Here's how the part is built. I have some questions about the finished solid (model axes, mm). A direction names the side the tool comes from. Round coordinates to 2 decimals unless told otherwise and drop trailing zeros. Loops run counter-clockwise (first coordinate to the right, second up) from the corner with the lowest first, then second, coordinate; pieces in that order, holes last. Notation, with made-up numbers: M 36,9 L 89,9 A26 ccw 89,45 Z; hole C 24.25,-28 d10. An arc over 180 degrees is marked long. Use a Markdown table: item, result.
Autodesk Inventor part; units mm, degrees
ref_plane "YZ Plane" through (0, 0, 0) normal (1, 0, 0) x (0, 1, 0)
ref_plane "XZ Plane" through (0, 0, 0) normal (0, 1, 0) x (-1, 0, 0)
ref_plane "XY Plane" through (0, 0, 0) normal (0, 0, 1) x (1, 0, 0)
sketch "スケッチ1" plane through (0, 0, 0) normal (0, 1, 0) x (-1, 0, 0)
  line L0 (0, 0) -> (53.8, 0)
  line L1 (53.8, 0) -> (53.8, -71.8)
  line L2 (53.8, -71.8) -> (0, -71.8)
  line L3 (0, -71.8) -> (0, 0)
  dimension "d0" = 53.8
  dimension "d1" = 71.8
extrude "押し出し1" add sketch "スケッチ1" along normal blind 10
sketch "スケッチ2" plane through (0, 10, 0) normal (0, 1, 0) x (1, 0, 0)
  line L0 (-53.8, 71.8) -> (-53.8, 0)
  line L1 (-53.8, 0) -> (0, 0)
  line L2 (-26.9, 0) -> (-26.9, 71.8)
  line L3 (0, 71.8) -> (-53.8, 71.8)
  line L4 (-53.8, 35.9) -> (0, 35.9)
  line L5 (0, 0) -> (0, 71.8)
  line L6 (-26.9, 35.9) -> (-37.05, 35.9)
  line L7 (-37.05, 35.9) -> (-37.05, 56.05)
  line L8 (-37.05, 56.05) -> (-26.9, 56.05)
  line L9 (-26.9, 56.05) -> (-26.9, 35.9)
  line L10 (-37.05, 35.9) -> (-37.05, 15.75)
  line L11 (-37.05, 15.75) -> (-26.9, 15.75)
  line L12 (-16.75, 35.9) -> (-16.75, 56.05)
  line L13 (-16.75, 56.05) -> (-26.9, 56.05)
  line L14 (-16.75, 35.9) -> (-16.75, 15.75)
  line L15 (-16.75, 15.75) -> (-26.9, 15.75)
  dimension "d7" = 20.15
  dimension "d8" = 10.15
extrude "押し出し2" add sketch "スケッチ2" along normal blind 40 contours L3 L2 L8 L7 L4 L0 | L4 L10 L11 L2 L1 L0 | L3 L5 L4 L12 L13 L2 | L2 L15 L14 L4 L5 L1
fillet "フィレット1" radius 5 4 edges at (0, 25, 0) (0, 25, -71.8) (-53.8, 25, -71.8) (-53.8, 25, 0)
sketch "スケッチ3" plane through (0, 0, -5) normal (1, 0, 0) x (0, 0, -1)
  line L0 (51.05, 50) -> (10.75, 50)
  line L1 (30.9, 50) -> (30.9, 0)
  line L2 (0, 0) -> (61.8, 0)
  line L3 (20.9, 50) -> (20.9, 0)
  line L4 (0, 50) -> (0, 0)
  line L5 (0, 10) -> (62, 10)
  line L6 (10.75, 10) -> (51.05, 10)
  point P0 (-5, 0)
  point P1 (20.9, 20)
  point P2 (20.9, 40)
  point P3 (40.9, 20)
  point P4 (40.9, 40)
  dimension "d12" = 10
  dimension "d13" = 10
  dimension "d14" = 10
  dimension "d15" = 20
hole "穴1" at (0, 20, -25.9) at (0, 40, -25.9) at (0, 40, -45.9) at (0, 20, -45.9) direction (-1, 0, 0) diameter 3.3 end through all
sketch "スケッチ4" plane through (0, 0, 0) normal (0, -1, 0) x (1, 0, 0)
  line L0 (-5, -71.8) -> (-48.8, -71.8)
  line L1 (-26.9, -71.8) -> (-26.9, 0)
  line L2 (-48.8, 0) -> (-5, 0)
  line L3 (-53.8, -66.8) -> (-53.8, -5)
  line L4 (-53.8, -35.9) -> (0, -35.9)
  line L5 (0, -5) -> (0, -66.8)
  point P0 (0, 0)
  point P1 (-26.9, -45.9)
  point P2 (-26.9, -25.9)
  dimension "d23" = 10
  dimension "d24" = 10
hole "穴2" at (-26.9, 0, -45.9) at (-26.9, 0, -25.9) direction (0, 1, 0) diameter 4.1 end through all
fillet "フィレット2" radius 1 4 edges at (-37.05, 50, -35.9) (-26.9, 50, -15.75) (-16.75, 50, -35.9) (-26.9, 50, -56.05)
sketch "スケッチ5" plane through (0, 0, 0) normal (0, -1, 0) x (1, 0, 0)
  circle A0 centre (-26.9, -25.9) radius 2.05
  circle A1 centre (-26.9, -45.9) radius 2.05
  line L0 (-26.9, -25.9) -> (-26.9, -45.9)
  line L1 (-26.9, -35.9) -> (-17.9, -35.9)
  line L2 (-17.9, -35.9) -> (-17.9, -42.9)
  line L3 (-17.9, -42.9) -> (-26.9, -42.9)
  line L4 (-26.9, -42.9) -> (-26.9, -35.9)
  line L5 (-17.9, -35.9) -> (-17.9, -28.9)
  line L6 (-17.9, -28.9) -> (-26.9, -28.9)
  line L7 (-35.9, -35.9) -> (-35.9, -42.9)
  line L8 (-35.9, -42.9) -> (-26.9, -42.9)
  line L9 (-35.9, -35.9) -> (-35.9, -28.9)
  line L10 (-35.9, -28.9) -> (-26.9, -28.9)
  point P0 (0, 0)
  dimension "d33" = 7
  dimension "d34" = 9
extrude "押し出し3" cut sketch "スケッチ5" against normal blind 10 contours L6 L5 L1 L0 | L0 L8 L7 L9 L10 | L1 L2 L3 L0
properties part number "framefixpart1"
1. Imagine slicing it at C-C, the plane y = 44. Write out the boundary of the cut face in (x, z), then the cut area to 3 significant figures.
Answer sheet:
| item | result |
|---|---|
| outline | M -53.8,-66.8 A5 ccw -48.8,-71.8 L -5,-71.8 A5 ccw 0,-66.8 L 0,-5 A5 ccw -5,0 L -48.8,0 A5 ccw -53.8,-5 Z; hole M -37.05,-56.05 L -16.75,-56.05 L -16.75,-15.75 L -37.05,-15.75 Z |
| area | 3,020 mm2 |
2. For pin 1 Ø3.5 at (x, z) = (-26.9, -45.9) entering from +Y; pin 2 Ø16 at (x, z) = (-25, -33.5) entering from +Y, each with a flat end and sliding along its axis, tell me the tip position at first contact or that it passes through.
Answer sheet:
| item | result |
|---|---|
| pin 1 | through |
| pin 2 | y = 10 |
3. Imagine slicing it at B-B, the plane x = -23. Write out the boundary of the cut face in (y, z), then the cut area to 3 significant figures.
Answer sheet:
| item | result |
|---|---|
| outline | M 0,-71.8 L 50,-71.8 L 50,-57.05 A1 ccw 49,-56.05 L 10,-56.05 L 10,-42.9 L 0,-42.9 Z; M 0,-28.9 L 10,-28.9 L 10,-15.75 L 49,-15.75 A1 ccw 50,-14.75 L 50,0 L 0,0 Z |
| area | 1,840 mm2 |
4. Imagine slicing it at A-A, the plane z = -45.9. State how many separate pieces and enclosed holes the cut face has, then the cut area to 3 significant figures.
Answer sheet:
| item | result |
|---|---|
| separate pieces | 6 |
| enclosed holes | 0 |
| area | 1,620 mm2 |
5. Which directions (+Z, -Z, +X, -X, +Y, -Y) give clear straight access to the entire face, cutting with the end or side of a thin tool? Please do faces 5 (the face through (-53.8, 25, -35)), 6 (the face through (-17.7, 10, -35.6)), 7 (the face through (-17.9, 5, -36)).
Answer sheet:
| item | result |
|---|---|
| face 5 | +Z, -Z, -X, +Y, -Y |
| face 6 | +Y |
| face 7 | +Y, -Y |
6. Imagine slicing it at D-D, the plane z = -30. Write out the boundary of the cut face in (x, y).
Answer sheet:
| item | result |
|---|---|
| outline | M -53.8,0 L -35.9,0 L -35.9,10 L -37.05,10 L -37.05,49 A1 ccw -38.05,50 L -53.8,50 Z; M -17.9,0 L 0,0 L 0,50 L -15.75,50 A1 ccw -16.75,49 L -16.75,10 L -17.9,10 Z |
7. We'd pull the mould along X, two halves only. Please class faces 1 (the face through (-27, 25, -71.8)), 2 (the face through (-25.081, 5.07, -26.846)), 3 (the face through (-16.75, 29, -36)), 4 (the face through (0, 25, -36)): +X half, -X half, draft (parallel to the pull), parting line (faces both ways), or undercut.
Answer sheet:
| item | result |
|---|---|
| face 1 | draft |
| face 2 | undercut |
| face 3 | undercut |
| face 4 | +X half |
8. I need wall thicknesses on probe 1 along Z at (x, y) = (-11, 40); probe 2 along Y at (x, z) = (-44, -45.9); probe 3 along X at (y, z) = (43, -50.5). Which ranges of each line are inside material? Lowest first, please. Write a range as from..to.
Answer sheet:
| item | result |
|---|---|
| probe 1 | -71.8..-47.55, -44.25..-27.55, -24.25..0 |
| probe 2 | 0..18.35, 21.65..38.35, 41.65..50 |
| probe 3 | -53.8..-37.05, -16.75..0 |
